from build123d import *

# Parameters (mm, degrees)
BOSS_EXTRU_1_DEPTH = 100
CONG_1_R           = 2
CONG_2_R           = 1


with BuildPart() as part:
    # Esquisse1 → Boss.-Extru.1 (new body)
    with BuildSketch(Plane.XY):
        Polygon((-11.5, 2.4), (11.5, 2.4), (11.5, 80), (40, 0), (-40, 0), (-11.5, 80), (-11.5, 60), (-9, 60), (-9, 50), (-11.5, 50), align=None)
        Polygon((13.9, 66.111581736), (13.9, 2.4), (36.597250994, 2.4), align=None, mode=Mode.SUBTRACT)
        Polygon((-13.9, 2.4), (-36.597250994, 2.4), (-13.9, 66.111581736), align=None, mode=Mode.SUBTRACT)
    extrude(amount=BOSS_EXTRU_1_DEPTH)

    # Congé1
    cong_1_edges = [part.edges().sort_by_distance(p)[0] for p in [
        (0, 0, 0),
        (11.5, 80, 50),
        (40, 0, 50),
        (-40, 0, 50),
        (-11.5, 80, 50),
        (-11.5, 2.4, 50),
        (11.5, 2.4, 50),
        (36.597250994, 2.4, 50),
        (13.9, 66.111581736, 50),
        (13.9, 2.4, 50),
        (0, 0, 100),
        (-13.9, 2.4, 50),
        (-13.9, 66.111581736, 50),
        (-36.597250994, 2.4, 50),
    ]]
    fillet(cong_1_edges, radius=CONG_1_R)

    # Congé2
    cong_2_edges = [part.edges().sort_by_distance(p)[0] for p in [
        (-11.5, 60, 50),
        (-9, 60, 50),
        (-9, 50, 50),
        (-11.5, 50, 50),
    ]]
    fillet(cong_2_edges, radius=CONG_2_R)


solid = part.part
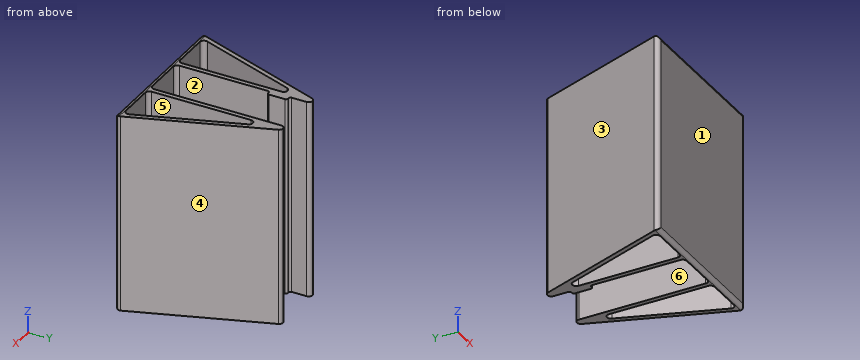
Part model, mm, in its own coordinate system. Face numbers are marked on the shaded views. A direction names the side the tool comes from. Coordinates: 2 decimals unless noted, no trailing zeros. Write each loop counter-clockwise with the first axis right and the second up, starting at its lowest first coordinate (ties: lowest second). Pieces come first, ordered by that corner, then holes. Notation, with made-up numbers: (87, -26) - (97, -26) arc R31 ccw to (97, 0) - close; hole circle Ø11 at (-21.75, -34.5). An arc over 180 degrees is marked (long way). Put each result on its own line as item: value.
1. Band-saw the part on A-A (z = 93). Give the number of separate pieces and of enclosed holes in the cut face, then the cut area to 3 significant figures.
Final values:
separate pieces: 1
enclosed holes: 2
area: 918 mm²
2. Band-saw the part on C-C (y = 40.5). Write the cut outline in (x, z).
Final values:
outline: (-25.57, 0) - (-23.02, 0) - (-23.02, 100) - (-25.57, 100) - close; (-13.9, 0) - (-11.5, 0) - (-11.5, 100) - (-13.9, 100) - close; (11.5, 0) - (13.9, 0) - (13.9, 100) - (11.5, 100) - close; (23.02, 0) - (25.57, 0) - (25.57, 100) - (23.02, 100) - close
3. Band-saw the part on B-B (x = 1). Write the cut outline in (y, z), then the cut area to 3 significant figures.
Final values:
outline: (0, 2) arc R2 ccw to (2, 0) - (2.4, 0) - (2.4, 100) - (2, 100) arc R2 ccw to (0, 98) - close
area: 238 mm²
4. Probe line 1 along X through (y, z) = (33.5, 13); line 2 along X through (y, z) = (12, 62) (3 decimals); line 3 along Y through (x, z) = (1, 79). List the from-to ranges inside material, lowest first. Write a range as [from, to].
Final values:
line 1: x = [-28.07, -25.52], [-13.9, -11.5], [11.5, 13.9], [25.52, 28.07]
line 2: x = [-35.725, -33.177], [-13.9, -11.5], [11.5, 13.9], [33.177, 35.725]
line 3: y = [0, 2.4]
5. Two-plate mould, pull along X, no slides. Class the marked faces 1, 2 and 3: +X half, -X half, draft (parallel to the pull), parting line (faces both ways), or undercut.
Final values:
face 1: draft
face 2: undercut
face 3: -X half
6. Band-saw the part on D-D (x = 29.5). Write the cut outline in (y, z), then the cut area to 3 significant figures.
Final values:
outline: (0, 2) arc R2 ccw to (2, 0) - (2.4, 0) - (2.4, 100) - (2, 100) arc R2 ccw to (0, 98) - close; (22.32, 0) - (29.47, 0) - (29.47, 100) - (22.32, 100) - close
area: 953 mm²
7. 3-axis set-ups, long thin cutter, end or side, ignore diameter. For the marked faces 4, 5 and 6: which of +Z, -Z, +X, -X, +Y, -Y reach the whole face in a straight line?
Final values:
face 4: +Z, -Z, +X, +Y
face 5: +Z, -Z
face 6: +Z, -Z, +Y
8. Flat gauge pins, fed straight in: pin 1 Ø6 at (y, z) = (63.5, 29) entering from +X; pin 2 Ø4 at (y, z) = (38, 85) entering from +X (3 decimals); pin 3 Ø25 at (y, z) = (30.5, 66) entering from -X. Where does each tip first touch, or does it go through?
Final values:
pin 1: stops at x = 18.45
pin 2: stops at x = 27.175
pin 3: stops at x = -33.59
